Here's how the part is built. I have some questions about the finished solid (model axes, mm). Round coordinates to 2 decimals unless told otherwise and drop trailing zeros. Write each loop counter-clockwise with the first axis right and the second up, starting at its lowest first coordinate (ties: lowest second). Pieces come first, ordered by that corner, then holes. Notation, with made-up numbers: M 65.5,4.25 L 75.5,4.25 A12 cw 75.5,9.25 Z; hole C 69,17.5 d5. An arc over 180 degrees is marked long. Use one line per item in the form item = value. Start each with the question number.
Q1. I need wall thicknesses on line 1 along X through (y, z) = (0.45, 11.96); line 2 along Z through (x, y) = (-78, 0.8); line 3 along Z through (x, y) = (-47.5, 0.1). Which ranges of each line are inside material? Lowest first, please. Write a range as from..to.
Q2. I want a section at A-A on x = -1.98. List the corners of the cut face in (y, z) for me, and give its area (3 significant figures).
Q3. I want a section at D-D on x = -32.48. List the corners of the cut face in (y, z) for me, and give its area (3 significant figures).
Q4. I want a section at C-C on x = -63.23. List the corners of the cut face in (y, z) for me.
Q5. I want a section at B-B on z = 25.5. List the corners of the cut face in (x, y) for me.
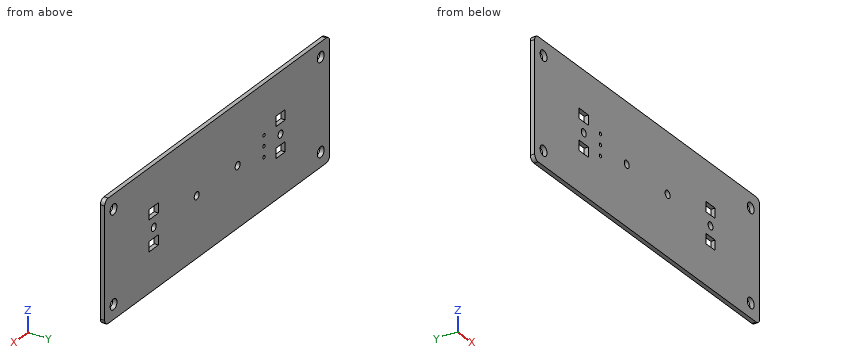
Autodesk Inventor part; units mm, degrees
ref_plane "YZ Plane" through (0, 0, 0) normal (1, 0, 0) x (0, 1, 0)
ref_plane "XZ Plane" through (0, 0, 0) normal (0, 1, 0) x (-1, 0, 0)
ref_plane "XY Plane" through (0, 0, 0) normal (0, 0, 1) x (1, 0, 0)
sketch "Boceto1" plane through (0, 0, 0) normal (0, 1, 0) x (-1, 0, 0)
  arc A0 (-1.27, 1.27) -> (0, 0) centre (0, 1.27) ccw
  line L0 (0, 0) -> (79.96, 0)
  arc A1 (79.96, 0) -> (81.23, 1.27) centre (79.96, 1.27) ccw
  line L1 (81.23, 1.27) -> (81.23, 27.73)
  arc A2 (81.23, 27.73) -> (79.96, 29) centre (79.96, 27.73) ccw
  line L2 (79.96, 29) -> (0, 29)
  arc A3 (0, 29) -> (-1.27, 27.73) centre (0, 27.73) ccw
  line L3 (-1.27, 27.73) -> (-1.27, 1.27)
  circle A4 centre (77.98, 3.5) radius 1.25
  circle A5 centre (1.98, 25.5) radius 1.25
  circle A6 centre (1.98, 3.5) radius 1.25
  circle A7 centre (77.98, 25.5) radius 1.25
  circle A8 centre (47.48, 14.5) radius 0.9
  circle A9 centre (32.48, 14.5) radius 0.9
  point P0 (0, 0)
extrude "Extrusión1" add sketch "Boceto1" along normal blind 1.04
sketch "Boceto3" plane through (0, 1.04, 0) normal (0, 1, 0) x (1, 0, 0)
  circle A0 centre (-63.23, -14.5) radius 0.9
  circle A1 centre (-16.73, -14.5) radius 0.9
  line L0 (-81.23, -1.27) -> (-81.23, -27.73)
  line L1 (0, 0) -> (-79.96, 0)
  line L2 (1.27, -27.73) -> (1.27, -1.27)
  line L3 (-79.96, -29) -> (0, -29)
  dimension "d15" = 1.8
  dimension "d16" = 1.8
  dimension "d17" = 18
  dimension "d18" = 14.5
  dimension "d19" = 18
  dimension "d20" = 14.5
hole "Agujero2" at (-63.23, 1.04, 14.5) at (-16.73, 1.04, 14.5) direction (0, -1, 0) diameter 1.8 end through all
sketch "Boceto4" plane through (0, 1.04, 0) normal (0, 1, 0) x (1, 0, 0)
  circle A0 centre (-57.13, -17.04) radius 0.4
  line L0 (-81.23, -1.27) -> (-81.23, -27.73)
  line L1 (-79.96, -29) -> (0, -29)
  circle A1 centre (-57.13, -14.5) radius 0.4
  circle A2 centre (-57.13, -11.96) radius 0.4
  line L2 (0, 0) -> (-79.96, 0)
  dimension "d28" = 0.8
  dimension "d29" = 24.1
  dimension "d30" = 11.96
  dimension "d31" = 0.8
  dimension "d32" = 0.8
  dimension "d33" = 11.96
  dimension "d34" = 2.54
  dimension "d35" = 2.54
hole "Agujero3" at (-57.13, 1.04, 17.04) at (-57.13, 1.04, 14.5) at (-57.13, 1.04, 11.96) direction (0, -1, 0) diameter 0.8 end through all
sketch "Boceto5" plane through (0, 0, 0) normal (0, -1, 0) x (1, 0, 0)
  line L0 (-15.03, 9.6) -> (-18.43, 9.6)
  line L1 (-18.43, 9.6) -> (-18.43, 12)
  line L2 (-18.43, 12) -> (-15.03, 12)
  line L3 (-15.03, 12) -> (-15.03, 9.6)
  line L4 (-79.96, 29) -> (0, 29)
  line L5 (1.27, 27.73) -> (1.27, 1.27)
  line L6 (-15.03, 17) -> (-18.43, 17)
  line L7 (-18.43, 17) -> (-18.43, 19.4)
  line L8 (-18.43, 19.4) -> (-15.03, 19.4)
  line L9 (-15.03, 19.4) -> (-15.03, 17)
  line L10 (0, 0) -> (-79.96, 0)
  line L11 (-61.53, 9.6) -> (-64.93, 9.6)
  line L12 (-64.93, 9.6) -> (-64.93, 12)
  line L13 (-64.93, 12) -> (-61.53, 12)
  line L14 (-61.53, 12) -> (-61.53, 9.6)
  line L15 (-81.23, 1.27) -> (-81.23, 27.73)
  line L16 (-61.53, 17) -> (-64.93, 17)
  line L17 (-64.93, 17) -> (-64.93, 19.4)
  line L18 (-64.93, 19.4) -> (-61.53, 19.4)
  line L19 (-61.53, 19.4) -> (-61.53, 17)
  dimension "d43" = 3.4
  dimension "d44" = 2.4
  dimension "d47" = 16.3
  dimension "d48" = 2.4
  dimension "d49" = 9.6
  dimension "d50" = 9.6
  dimension "d51" = 3.4
  dimension "d52" = 2.4
  dimension "d53" = 9.6
  dimension "d54" = 16.3
  dimension "d55" = 3.4
  dimension "d56" = 2.4
  dimension "d57" = 16.3
  dimension "d58" = 9.6
extrude "Extrusión2" cut sketch "Boceto5" against normal through all
sketch "Boceto6" plane through (0, 0, 0) normal (0, -1, 0) x (1, 0, 0)
  point P0 (0, 0)
properties part number "Interstage A"
Reported:
q1.line_1 = -81.23..-64.93, -61.53..-57.53, -56.73..-18.43, -15.03..1.27
q1.line_2 = 0..2.25, 4.75..24.25, 26.75..29
q1.line_3 = 0..13.6, 15.4..29
q2.outline = M 0,0 L 1.04,0 L 1.04,2.25 L 0,2.25 Z; M 0,4.75 L 1.04,4.75 L 1.04,24.25 L 0,24.25 Z; M 0,26.75 L 1.04,26.75 L 1.04,29 L 0,29 Z
q2.area = 25.0 mm^2
q3.outline = M 0,0 L 1.04,0 L 1.04,13.6 L 0,13.6 Z; M 0,15.4 L 1.04,15.4 L 1.04,29 L 0,29 Z
q3.area = 28.3 mm^2
q4.outline = M 0,0 L 1.04,0 L 1.04,9.6 L 0,9.6 Z; M 0,12 L 1.04,12 L 1.04,13.6 L 0,13.6 Z; M 0,15.4 L 1.04,15.4 L 1.04,17 L 0,17 Z; M 0,19.4 L 1.04,19.4 L 1.04,29 L 0,29 Z
q5.outline = M -81.23,0 L -79.23,0 L -79.23,1.04 L -81.23,1.04 Z; M -76.73,0 L -3.23,0 L -3.23,1.04 L -76.73,1.04 Z; M -0.73,0 L 1.27,0 L 1.27,1.04 L -0.73,1.04 Z
